Here's how the part is built. I have some questions about the finished solid (model axes, mm). Face numbers are marked on the shaded views. A direction names the side the tool comes from. Give positions to 0.01 mm unless a question says otherwise; leave off trailing zeros. Order: outer loops, then holes, each group sorted by start corner. A loop starts at its lowest first (then second) coordinate and runs counter-clockwise, first axis right, second up. Notation, with made-up numbers: (44, -20.75) -> (55, -20.75) arc R19 ccw to (55, 13.25) -> close; hole circle Ø8 at (3, -38). An arc over 180 degrees is marked (long way). Write each question's results on one line, items separated by ' | '. Start each with the question number.
Q1. Imagine slicing it at C-C, the plane y = -20. Please give me the cut outline in (x, z), then the cut area to 3 significant figures.
Q2. Thinking about a two-plate mould opening in X: for the marked faces 4, 5, 6 and 7, which applies, pulls with the +X half, pulls with the -X half, needs draft (parallel to the pull), parting line crosses it, or undercut?
Q3. I need wall thicknesses on line 1 along Y through (x, z) = (-16, 1.85); line 2 along Z through (x, y) = (16, 28); line 3 along X through (y, z) = (-20, 1.7). Which ranges of each line are inside material? Lowest first, please. Write a range as [from, to].
Q4. Imagine slicing it at D-D, the plane y = 15. Please give me the cut outline in (x, z).
Q5. For the marked faces 1, 2 and 3, which set-ups out of +Z, -Z, +X, -X, +Y, -Y let a thin tool reach every point of the face, with its end or its side?
Q6. Imagine slicing it at B-B, the plane x = 16. Please give me the cut outline in (y, z).
Q7. I'm going to push flat-ended pins straight in: pin 1 (2 mm diameter, centred on x = 23, z = 24, fed in from +Y); pin 2 (5 mm diameter, centred on x = -16, y = -20, fed in from -Z); pin 3 (10 mm diameter, centred on x = 6, z = 24, fed in from -Y); pin 4 (3 mm diameter, centred on x = 0.5, y = -13.5, fed in from +Z). Where does each tip first touch, or does it pass through?
Q8. Imagine slicing it at A-A, the plane z = 13. Please give me the cut outline in (x, y), then the cut area to 3 significant figures.
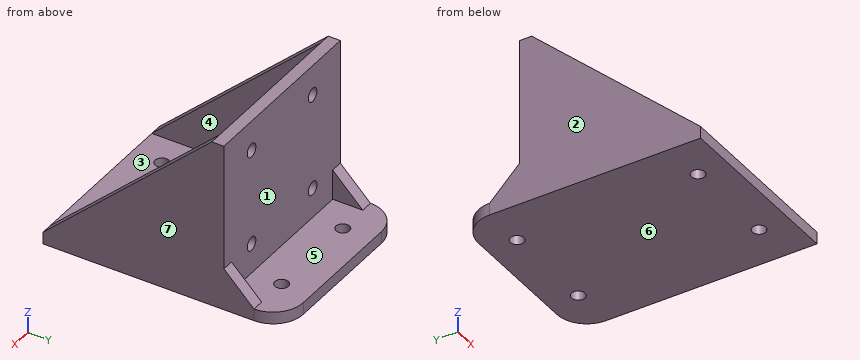
```python
from build123d import *

# Parameters (mm, degrees)
F0_W      = 53
F0_H      = 60
F1_DEPTH  = 4
F2_W      = 53
F2_H      = 4
F3_DEPTH  = 52
F4_R      = 2.25
F5_DEPTH  = 56.001
F6_R      = 2.25
F7_DEPTH  = 60.001
F9_DEPTH  = 4
F11_DEPTH = 4
F12_W     = 61
F12_H     = 4
F13_DEPTH = 20
F14_R     = 2.25
F15_DEPTH = 4.001
F16_R     = 10


# Not quite as in the source:
# - a feature names something its author has since deleted; it is built from what else it names


with BuildPart() as f1:
    # F0 (on Top) → F1 (new body)
    with BuildSketch(Plane.XY):
        Rectangle(F0_W, F0_H)
    extrude(amount=F1_DEPTH)

    # F2 (on face) → F3 (join)
    with BuildSketch(Plane.XY.offset(4)):
        with Locations((0, 28)):
            Rectangle(F2_W, F2_H)
    extrude(amount=F3_DEPTH)

    # F4 (on face) → F5 (cut, through all)
    with BuildSketch(Plane(origin=(0, 0, 0), x_dir=(1, 0, 0), z_dir=(0, 0, -1))):
        with Locations((-16, 20)):
            Circle(F4_R)
        with Locations((16, 20)):
            Circle(F4_R)
    extrude(amount=-F5_DEPTH, mode=Mode.SUBTRACT)

    # F6 (on face) → F7 (cut, through all)
    with BuildSketch(Plane(origin=(0, 30, 0), x_dir=(-1, 0, 0), z_dir=(0, 1, 0))):
        with Locations((-16, 14)):
            Circle(F6_R)
        with Locations((-16, 46)):
            Circle(F6_R)
        with Locations((16, 14)):
            Circle(F6_R)
        with Locations((16, 46)):
            Circle(F6_R)
    extrude(amount=-F7_DEPTH, mode=Mode.SUBTRACT)

    # F8 (on face) → F9 (join)
    with BuildSketch(Plane.YZ.offset(26.5)):
        Polygon((30, 14), (30, 56), (26, 56), (-30, 4), (-30, 0), (30, 0), (30, 4), align=None)
        Polygon((40, 4), (30, 14), (30, 4), align=None)
    extrude(amount=F9_DEPTH)

    # F10 (on face) → F11 (join)
    with BuildSketch(Plane(origin=(-26.5, 0, 0), x_dir=(0, -1, 0), z_dir=(-1, 0, 0))):
        Polygon((-26, 56), (-30, 56), (-30, 14), (-30, 4), (-30, 0), (30, 0), (30, 4), align=None)
        Polygon((-30, 4), (-30, 14), (-40, 4), align=None)
    extrude(amount=F11_DEPTH)

    # F12 (on face) → F13 (join)
    with BuildSketch(Plane(origin=(0, 30, 0), x_dir=(-1, 0, 0), z_dir=(0, 1, 0))):
        with Locations((0, 2)):
            Rectangle(F12_W, F12_H)
    extrude(amount=F13_DEPTH)

    # F14 (on face) → F15 (cut, through all)
    with BuildSketch(Plane.XY.offset(4)):
        with Locations((16, 40)):
            Circle(F14_R)
        with Locations((-16, 40)):
            Circle(F14_R)
    extrude(amount=-F15_DEPTH, mode=Mode.SUBTRACT)

    # F16
    f16_edges = [f1.edges().sort_by_distance(p)[0] for p in [
        (30.5, 50, 2),
        (-30.5, 50, 2),
    ]]
    fillet(f16_edges, radius=F16_R)


solid = f1.part
```
Geometry check:
1) outline: (-30.5, 0) -> (-18.25, 0) -> (-18.25, 4) -> (-26.5, 4) -> (-26.5, 13.29) -> (-30.5, 13.29) -> close; (-13.75, 0) -> (13.75, 0) -> (13.75, 4) -> (-13.75, 4) -> close; (18.25, 0) -> (30.5, 0) -> (30.5, 13.29) -> (26.5, 13.29) -> (26.5, 4) -> (18.25, 4) -> close | area: 282 mm²
2) face 4: undercut | face 5: undercut | face 6: needs draft | face 7: pulls with the +X half
3) line 1: [-30, -22.25], [-17.75, 37.75], [42.25, 50] | line 2: [0, 11.75], [16.25, 43.75], [48.25, 56] | line 3: [-30.5, -18.25], [-13.75, 13.75], [18.25, 30.5]
4) outline: (-30.5, 0) -> (30.5, 0) -> (30.5, 45.79) -> (26.5, 45.79) -> (26.5, 4) -> (-26.5, 4) -> (-26.5, 45.79) -> (-30.5, 45.79) -> close
5) face 1: +Z, +Y | face 2: +Z, -Z, -X, +Y, -Y | face 3: +Z, -Y
6) outline: (-30, 0) -> (-22.25, 0) -> (-22.25, 4) -> (-30, 4) -> close; (-17.75, 0) -> (37.75, 0) -> (37.75, 4) -> (30, 4) -> (30, 11.75) -> (26, 11.75) -> (26, 4) -> (-17.75, 4) -> close; (26, 16.25) -> (30, 16.25) -> (30, 43.75) -> (26, 43.75) -> close; (26, 48.25) -> (30, 48.25) -> (30, 56) -> (26, 56) -> close; (42.25, 0) -> (50, 0) -> (50, 4) -> (42.25, 4) -> close
7) pin 1: y = 30 | pin 2: z = 0 | pin 3: y = 26 | pin 4: z = 4
8) outline: (-30.5, -20.31) -> (-26.5, -20.31) -> (-26.5, 26) -> (-18.02, 26) -> (-18.02, 30) -> (-26.5, 30) -> (-26.5, 31) -> (-30.5, 31) -> close; (-13.98, 26) -> (13.98, 26) -> (13.98, 30) -> (-13.98, 30) -> close; (18.02, 26) -> (26.5, 26) -> (26.5, -20.31) -> (30.5, -20.31) -> (30.5, 31) -> (26.5, 31) -> (26.5, 30) -> (18.02, 30) -> close | area: 590 mm²
